```python
from build123d import *

# Parameters (mm, degrees)
SKETCH1_W           = 20
SKETCH1_H           = 80
BOSS_EXTRUDE1_DEPTH = 5
SHELL1_T            = -2
FILLET1_R           = 3
FILLET2_R           = 3
FILLET3_R           = 3
FILLET4_R           = 3
FILLET5_R           = 3
FILLET6_R           = 3
FILLET7_R           = 3
FILLET8_R           = 3
SKETCH2_W           = 6
SKETCH2_H           = 5
BOSS_EXTRUDE2_DEPTH = 6
SKETCH3_R           = 1.425
CUT_EXTRUDE1_DEPTH  = 4


with BuildPart() as part:
    # Sketch1 → Boss-Extrude1 (new body)
    with BuildSketch(Plane(origin=(0, 0, 0), x_dir=(1, 0, 0), z_dir=(0, 1, 0))):
        with Locations((10, 40)):
            Rectangle(SKETCH1_W, SKETCH1_H)
    extrude(amount=BOSS_EXTRUDE1_DEPTH)

    # Shell1
    shell1_openings = [part.faces().sort_by_distance(p)[0] for p in [
        (10, 5, -40),
    ]]
    offset(amount=SHELL1_T, openings=shell1_openings, kind=Kind.INTERSECTION)

    # Fillet1
    fillet1_edges = [part.edges().sort_by_distance(p)[0] for p in [
        (20, 2.5, 0),
    ]]
    fillet(fillet1_edges, radius=FILLET1_R)

    # Fillet2
    fillet2_edges = [part.edges().sort_by_distance(p)[0] for p in [
        (0, 2.5, 0),
    ]]
    fillet(fillet2_edges, radius=FILLET2_R)

    # Fillet3
    fillet3_edges = [part.edges().sort_by_distance(p)[0] for p in [
        (20, 2.5, -80),
    ]]
    fillet(fillet3_edges, radius=FILLET3_R)

    # Fillet4
    fillet4_edges = [part.edges().sort_by_distance(p)[0] for p in [
        (0, 2.5, -80),
    ]]
    fillet(fillet4_edges, radius=FILLET4_R)

    # Fillet5
    fillet5_edges = [part.edges().sort_by_distance(p)[0] for p in [
        (2, 3.5, -2),
    ]]
    fillet(fillet5_edges, radius=FILLET5_R)

    # Fillet6
    fillet6_edges = [part.edges().sort_by_distance(p)[0] for p in [
        (18, 3.5, -2),
    ]]
    fillet(fillet6_edges, radius=FILLET6_R)

    # Fillet7
    fillet7_edges = [part.edges().sort_by_distance(p)[0] for p in [
        (2, 3.5, -78),
    ]]
    fillet(fillet7_edges, radius=FILLET7_R)

    # Fillet8
    fillet8_edges = [part.edges().sort_by_distance(p)[0] for p in [
        (18, 3.5, -78),
    ]]
    fillet(fillet8_edges, radius=FILLET8_R)

    # Sketch2 → Boss-Extrude2 (add)
    with BuildSketch(Plane.ZY):
        with Locations((-40, 2.5)):
            Rectangle(SKETCH2_W, SKETCH2_H)
    extrude(amount=BOSS_EXTRUDE2_DEPTH)

    # Sketch3 → Cut-Extrude1 (cut)
    with BuildSketch(Plane.ZY.offset(6)):
        with Locations((-40, 2.5)):
            Circle(SKETCH3_R)
    extrude(amount=-CUT_EXTRUDE1_DEPTH, mode=Mode.SUBTRACT)


solid = part.part
```
The model under review builds one solid part; all positions refer to its coordinate system, in mm. A direction names the side the tool comes from. Coordinates: 2 decimals unless noted, no trailing zeros. Write each loop counter-clockwise with the first axis right and the second up, starting at its lowest first coordinate (ties: lowest second). Pieces come first, ordered by that corner, then holes.
1) Machinability: for faces 1 (the face through (10, 3, -78)), 2 (the face through (-4.028, 1.954, -38.684)), 3 (the face through (0, 2, -60)), which of the approach directions +Z, -Z, +X, -X, +Y, -Y give a long, thin tool a straight path to every point of the face, cutting with its end or side? Answer none if there is none.
2) We need section B-B on x = 14.25. State the section outline as (y, z) points, then the cut area to 3 significant figures.
3) To check wall thickness, follow probe 1 along Y at (x, z) = (-3.55, -40) (3 decimals); probe 2 along X at (y, z) = (4.2, -58.5); probe 3 along Z at (x, y) = (10, 3.6). State the ranges of each line that lie inside material, in increasing order.
4) We need section A-A on z = -46.5. State the section outline as (x, y) points.
5) Clearance check with flat-ended pins moving along their axes: pin 1 Ø2.5 at (y, z) = (1.5, -19) entering from -X; pin 2 Ø2.5 at (x, y) = (-1.5, 1.5) entering from -Z; pin 3 Ø8 at (x, z) = (11.5, -22) entering from +Y. State where each tip first meets the part, or that it passes through.
6) The part is to be moulded in two halves that separate along Z. For faces 4 (the face through (10, 2, -80)), 5 (the face through (2.9, 3.48, -2.86)), 6 (the face through (2, 3, -40)), 7 (the face through (19.1, 2.54, -0.86)), say which applies: pulls with the +Z half, pulls with the -Z half, needs draft (parallel to the pull), parting line crosses it, or undercut.
Answer list:
1. face 1: +Y
1. face 2: -X
1. face 3: -Z, -X, +Y, -Y
2. outline: (0, -80) - (5, -80) - (5, -78) - (2, -78) - (2, -2) - (5, -2) - (5, 0) - (0, 0) - close
2. area: 172 mm2
3. probe 1: y = 0 to 1.075, 3.925 to 5
3. probe 2: x = 0 to 2, 18 to 20
3. probe 3: z = -80 to -78, -2 to 0
4. outline: (0, 0) - (20, 0) - (20, 5) - (18, 5) - (18, 2) - (2, 2) - (2, 5) - (0, 5) - close
5. pin 1: stops at x = 0
5. pin 2: stops at z = -43
5. pin 3: stops at y = 2
6. face 4: pulls with the -Z half
6. face 5: undercut
6. face 6: undercut
6. face 7: pulls with the +Z half
